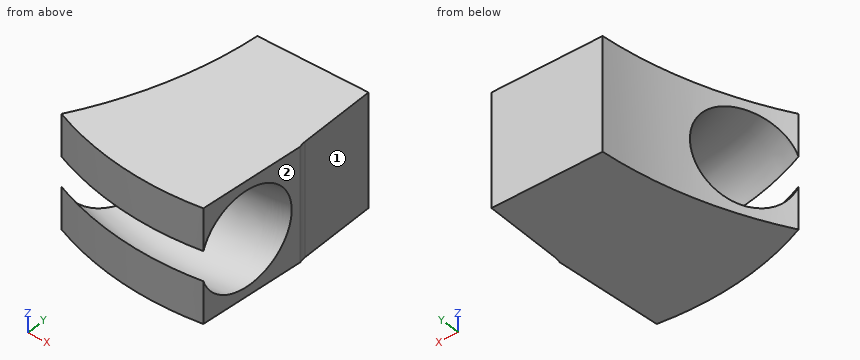
Autodesk Inventor part; units mm, degrees
ref_plane "Work Plane1" through (-5.5192, -8.9325, 0) normal (0.85071, -0.5256353, 0) x (0.5256353, 0.85071, 0)
ref_plane "YZ Plane" through (0, 0, 0) normal (1, 0, 0) x (0, 1, 0)
ref_plane "XZ Plane" through (0, 0, 0) normal (0, 1, 0) x (-1, 0, 0)
sketch "Block1" plane through (0, 0, 0) normal (0, 0, 1) x (1, 0, 0)
  arc A0 (19.4993, -13.8282) -> (19.4817, -14.1291) centre (20.4774, -14.0361) ccw construction
  line L0 (19.4993, -13.8282) -> (20.7824, -7.7917) construction
  arc A1 (21.6494, -6.5302) -> (20.7824, -7.7917) centre (22.7387, -8.2075) ccw construction
  line L1 (21.6494, -6.5302) -> (21.8911, -6.3732) construction
  arc A2 (21.8911, -6.3732) -> (16.2026, -4.7141) centre (18.9149, -5.9962) ccw construction
  arc A3 (16.1932, -4.631) -> (16.2026, -4.7141) centre (16.693, -4.6165) ccw construction
  arc A4 (16.2, -5.1) -> (16.1932, -4.631) centre (0, -5.1) ccw construction
  arc A5 (11.587, -16.123) -> (16.2, -5.1) centre (0, -4.7972) ccw construction
  arc A6 (11.587, -16.123) -> (18.1044, -18.4699) centre (18.9149, -5.9962) ccw construction
  line L2 (19.4817, -14.1291) -> (18.1044, -18.4699) construction
  circle A7 centre (18.9149, -5.9962) radius 1 construction
  arc A8 (21.7954, -6.3313) -> (16.3027, -4.7365) centre (18.9149, -5.9962) ccw
  arc A9 (21.7954, -6.3313) -> (20.6845, -7.7709) centre (22.7387, -8.2075) ccw
  line L3 (20.6845, -7.7709) -> (19.4014, -13.8074)
  arc A10 (19.4014, -13.8074) -> (19.3804, -14.1177) centre (20.4774, -14.0361) ccw
  line L4 (19.3804, -14.1177) -> (18.0329, -18.3647)
  arc A11 (11.7396, -16.1093) -> (18.0329, -18.3647) centre (18.9149, -5.9962) ccw
  arc A12 (11.7396, -16.1093) -> (16.3027, -4.7365) centre (0, -4.7972) ccw
  line L5 (15.5605, -9.6605) -> (20.0788, -10.6209)
  point P0 (17.4447, -9.0721)
  dimension "d0" = 0.1
  dimension "d1" = 8
sketch "Sketch1" plane through (0, 0, 0) normal (0, 0, 1) x (1, 0, 0)
  circle A0 centre (0, 0) radius 10.5 construction
  line L0 (-5.5192, -8.9325) -> (1.2791, -13.1329) construction
  arc A1 (2.2, -7.5394) -> (2.2454, -7.8373) centre (3.2, -7.5394) ccw construction
  line L1 (2.2, -7.5394) -> (2.2, -1.368) construction
  arc A2 (2.7858, 0.0462) -> (2.2, -1.368) centre (4.2, -1.368) ccw construction
  line L2 (2.7858, 0.0462) -> (2.9896, 0.25) construction
  arc A3 (2.9896, 0.25) -> (-2.9195, 0.6901) centre (0, 0) ccw construction
  arc A4 (-2.946, 0.7695) -> (-2.9195, 0.6901) centre (-2.4602, 0.8876) ccw construction
  arc A5 (-2.8419, 0.3121) -> (-2.946, 0.7695) centre (-18.6879, -3.0561) ccw construction
  arc A6 (-5.0623, -11.4291) -> (-2.8419, 0.3121) centre (-18.7508, -2.7598) ccw construction
  arc A7 (-5.0623, -11.4291) -> (1.8007, -12.3696) centre (0, 0) ccw construction
  line L3 (2.2454, -7.8373) -> (1.8007, -12.3696) construction
  circle A8 centre (0, 0) radius 1 construction
  arc A9 (2.8873, 0.2711) -> (-2.817, 0.689) centre (0, 0) ccw
  arc A10 (2.8873, 0.2711) -> (2.1, -1.368) centre (4.2, -1.368) ccw
  line L4 (2.1, -1.368) -> (2.1, -7.5394)
  arc A11 (2.1, -7.5394) -> (2.144, -7.8473) centre (3.2, -7.5394) ccw
  line L5 (2.144, -7.8473) -> (1.7089, -12.2817)
  arc A12 (-4.9158, -11.384) -> (1.7089, -12.2817) centre (0, 0) ccw
  arc A13 (-4.9158, -11.384) -> (-2.817, 0.689) centre (-18.7508, -2.7598) ccw
  line L6 (-2.5192, -4.2817) -> (2.1, -4.2817)
  dimension "d4" = 21
  dimension "d5" = 3
extrude "Extrusion1" add sketch "Sketch1" along normal mid plane 4.8 contours L6 L4 A11 L5 A12 A13
ref_plane "Work Plane1" through (-5.5192, -8.9325, 0) normal (0.85071, -0.5256353, 0) x (0.5256353, 0.85071, 0)
sketch "Sketch2" plane through (-5.5192, -8.9325, 0) normal (0.85071, -0.5256353, 0) x (0.5256353, 0.85071, 0)
  circle A0 centre (0, 0) radius 2
  line L0 (10.5, -2.8) -> (10.5, 2.8)
  point P0 (10.5, 0)
  dimension "d6" = 4
revolve "Revolution1" cut sketch "Sketch2" angle 360 about axis through (0, 0, 0) along (0, 0, 1)
properties part number "ORingToolA"
Geometry: final body of the model. Coordinates: model frame, mm. Face numbers are marked on the shaded views. A direction names the side the tool comes from. Round coordinates to 2 decimals unless told otherwise and drop trailing zeros. Write each loop counter-clockwise with the first axis right and the second up, starting at its lowest first coordinate (ties: lowest second). Pieces come first, ordered by that corner, then holes. Notation, with made-up numbers: (3.25, 46) -> (55.25, 46) arc R21 ccw to (55.25, 63) -> close; hole circle Ø10 at (85.25, -20). An arc over 180 degrees is marked (long way). Return JSON: item names as keys, results as strings.
Q1. Section B-B on y = -6. Return the cut outline in (x, z).
From the geometry:
{"outline": "(-2.77, -2.4) -> (2.1, -2.4) -> (2.1, 2.4) -> (-2.77, 2.4) -> close"}
Q2. Section A-A on y = -7.75. Return the cut outline in (x, z), and give its area (3 significant figures).
From the geometry:
{"outline": "(-3.23, -2.4) -> (2.12, -2.4) -> (2.12, 2.4) -> (-3.23, 2.4) -> close", "area": "25.7 mm2"}
Q3. First-contact query: pin 1 Ø2.5 at (y, z) = (-6, 0) entering from +X. Flat tip, straight axial feed; report the tip coordinate or a pass-through.
From the geometry:
{"pin 1": "x = 2.1"}
Q4. Ray query, line 1 (Y direction, x = 1.25, z = -1.3); line 2 (Z direction, x = -3.75, y = -10.5); line 3 (Y direction, x = -1.5, z = -1.8). Return the intervals inside material, ascending.
From the geometry:
{"line 1": "-12.34 to -11.95, -8.89 to -4.28", "line 2": "-2.4 to -1.89, 1.89 to 2.4", "line 3": "-12.31 to -11.27, -9.51 to -4.28"}
Q5. Set-up query: the marked faces 1 and 2. Return all of +Z, -Z, +X, -X, +Y, -Y with unobstructed straight access to the full face (end or side cutting, diameter ignored); none if empty.
From the geometry:
{"face 1": "+Z, -Z, +X, +Y", "face 2": "+Z, -Z, +X, -Y"}
